Source: CAD feature listing. Evaluate the final solid. Frame: model axes, mm. Face numbers are marked on the shaded views. A direction names the side the tool comes from. Give positions to 0.01 mm unless a question says otherwise; leave off trailing zeros. Order: outer loops, then holes, each group sorted by start corner. A loop starts at its lowest first (then second) coordinate and runs counter-clockwise, first axis right, second up. Notation, with made-up numbers: M 87.25,-5.75 L 120.25,-5.75 A26 cw 120.25,32.25 Z; hole C 0.5,-4.5 d9. An arc over 180 degrees is marked long. Answer in a Markdown table with one row per item. Add a question column.
(1) Section query A-A, the plane z = 0. Return loops of the section in (x, y), plus the area to 3 significant figures.
(2) Pin query (flat end, axial travel): P1, Ø3, axis at y = 1, z = -2.5, coming from the -X side; P2, Ø5, axis at x = 0, z = 0, coming from the +Y side; P3, Ø2, axis at x = 0, y = 3, coming from the -Z side; P4, Ø2, axis at y = 2.5, z = -2.5, coming from the -X side. Return the tip coordinate at first contact, or that it passes through.
(3) Set-up query: the marked faces 1, 2 and 3. Return all of +Z, -Z, +X, -X, +Y, -Y with unobstructed straight access to the full face (end or side cutting, diameter ignored); none if empty.
(4) Material intervals for line 1 along X through (y, z) = (3.85, 0); line 2 along Z through (x, y) = (-4.5, 2.8); line 3 along X through (y, z) = (0.85, 2.25), sorted ascending.
(5) Section query C-C, the plane y = 0.8. Return loops of the section in (x, z).
(6) Section query B-B, the plane x = -2.75. Return loops of the section in (y, z).
(7) Section query D-D, the plane x = 0. Return loops of the section in (y, z).
(8) Mould query, pull axis X, two halves, no side actions, for the marked faces 4, 5, 6 and 7. Classes: pulls with the +X half, pulls with the -X half, needs draft (parallel to the pull), parting line crosses it, or undercut.
from build123d import *

# Parameters (mm, degrees)
CROQUIS1_R              = 3
SALIENTE_EXTRUIR1_DEPTH = 5
CORTAR_EXTRUIR1_START   = -5
CORTAR_EXTRUIR1_DEPTH   = 5
CORTAR_EXTRUIR2_DEPTH   = 10


# Read off the part's stored shape, not the designer's step: Cortar-Extruir1
with BuildPart() as part:
    # Croquis1 → Saliente-Extruir1 (new body)
    with BuildSketch(Plane(origin=(0, 0, 0), x_dir=(1, 0, 0), z_dir=(0, 1, 0))):
        with BuildLine():
            Line((-5, 7), (-5, 3))
            Line((-5, 3), (-4, 3))
            ThreePointArc((-4, 3), (0, -5), (4, 3))
            Line((4, 3), (5, 3))
            Line((5, 3), (5, 7))
            ThreePointArc((5, 7), (0, 5), (-5, 7))
        make_face()
        with Locations(Location((0, 0, 0), (0, 0, 270))):
            Circle(CROQUIS1_R, mode=Mode.SUBTRACT)
    extrude(amount=SALIENTE_EXTRUIR1_DEPTH)

    # Cortar-Extruir1 outline → Cortar-Extruir1 (cut)
    with BuildSketch(Plane(origin=(0, 5, 0), x_dir=(1, 0, 0), z_dir=(0, 1, 0)).offset(CORTAR_EXTRUIR1_START)):
        with BuildLine():
            Line((-2.974891432, -0.387325401), (-2.5, -4.330127019))
            ThreePointArc((-2.5, -4.330127019), (0, -5), (2.5, -4.330127019))
            Line((2.5, -4.330127019), (2.974891432, -0.387325401))
            ThreePointArc((2.974891432, -0.387325401), (0, -3), (-2.974891432, -0.387325401))
        make_face()
    extrude(amount=CORTAR_EXTRUIR1_DEPTH, mode=Mode.SUBTRACT)

    # Croquis3 → Cortar-Extruir2 (cut)
    with BuildSketch(Plane(origin=(0, 5, 0), x_dir=(1, 0, 0), z_dir=(0, 1, 0))):
        Polygon((4, 3), (5, 4.732050808), (5, 3), align=None)
        Polygon((-4, 3), (-5, 4.732050808), (-5, 3), align=None)
    extrude(amount=-CORTAR_EXTRUIR2_DEPTH, mode=Mode.SUBTRACT)


solid = part.part
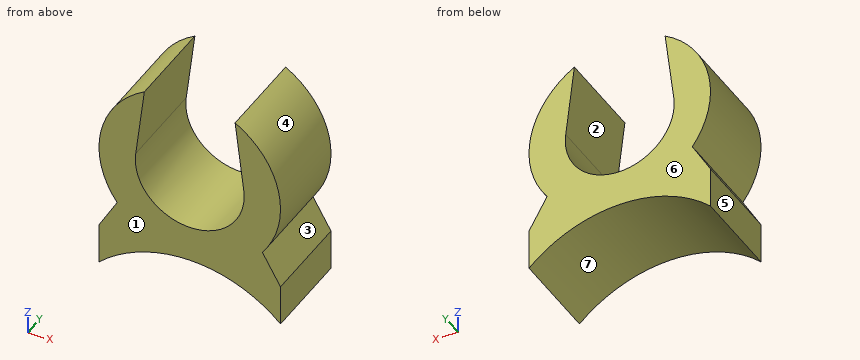
Values follow:
| question | item | result |
|---|---|---|
| 1 | outline | M -5,0 L -3,0 L -3,5 L -5,5 Z; M 3,0 L 5,0 L 5,5 L 3,5 Z |
| 1 | area | 20.0 mm² |
| 2 | P1 | stops at x = -4.9 |
| 2 | P2 | passes through |
| 2 | P3 | stops at z = -5.07 |
| 2 | P4 | stops at x = -4.77 |
| 3 | face 1 | +Z, -Z, +X, -X, -Y |
| 3 | face 2 | +Y, -Y |
| 3 | face 3 | +X, +Y, -Y |
| 4 | line 1 | x = -5 to -3, 3 to 5 |
| 4 | line 2 | z = -6.57 to -3.87, -2.18 to 2.18 |
| 4 | line 3 | x = -4.47 to -2.75, 2.75 to 4.47 |
| 5 | outline | M -5,-7 A7.25 cw 5,-7 L 5,-4.73 L 4,-3 A5 ccw 2.5,4.33 L 2.97,0.39 A3 cw long -2.97,0.39 L -2.5,4.33 A5 ccw -4,-3 L -5,-4.73 Z |
| 6 | outline | M 0,-5.54 L 5,-5.54 L 5,-1.2 L 0,-1.2 Z; M 0,2.25 L 5,2.25 L 5,4.18 L 0,4.18 Z |
| 7 | outline | M 0,-5 L 5,-5 L 5,-3 L 0,-3 Z |
| 8 | face 4 | pulls with the +X half |
| 8 | face 5 | pulls with the -X half |
| 8 | face 6 | needs draft |
| 8 | face 7 | undercut |
